Read the model definition and answer for the solid it produces. Units are mm, in the model's axes. Give positions to 0.01 mm unless a question says otherwise; leave off trailing zeros. Order: outer loops, then holes, each group sorted by start corner. A loop starts at its lowest first (then second) coordinate and runs counter-clockwise, first axis right, second up. Notation, with made-up numbers: (78, 32.25) -> (94, 32.25) arc R24 cw to (94, 53.25) -> close; hole circle Ø7 at (-35.75, 72). An arc over 180 degrees is marked (long way). One line per item, written item: value. Start each with the question number.
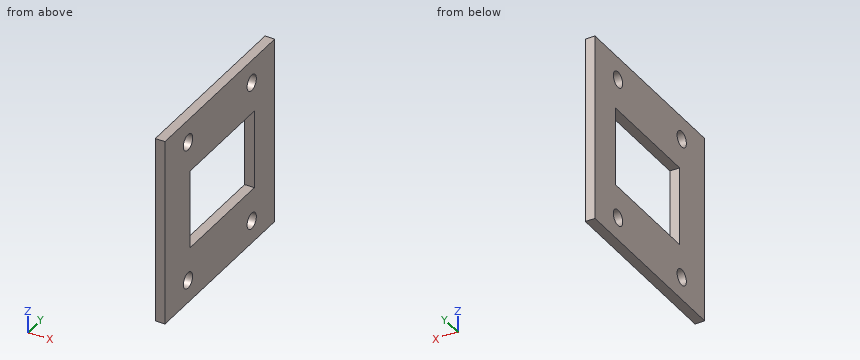
from build123d import *

# Parameters (mm, degrees)
SKETCH1_W           = 61.8
SKETCH1_H           = 62
BOSS_EXTRUDE1_DEPTH = 3.2
CUT_EXTRUDE1_REACH  = 5.2
SKETCH2_W           = 26
SKETCH2_H           = 36.3
CUT_EXTRUDE2_REACH  = 5.2
SKETCH3_R           = 2.625


with BuildPart() as part:
    # Sketch1 → Boss-Extrude1 (new body)
    with BuildSketch(Plane(origin=(0, 0, 0), x_dir=(0, 0, -1), z_dir=(1, 0, 0))):
        with Locations((30.9, 31)):
            Rectangle(SKETCH1_W, SKETCH1_H)
    extrude(amount=BOSS_EXTRUDE1_DEPTH)

    # Sketch2 → Cut-Extrude1 (cut, up to next)
    with BuildSketch(Plane(origin=(3.2, 0, 0), x_dir=(0, 0, -1), z_dir=(1, 0, 0)), mode=Mode.PRIVATE) as cut_extrude1_sk1:
        with Locations((30.9, 32.35)):
            Rectangle(SKETCH2_W, SKETCH2_H)
    cut_extrude1_tool1 = extrude(cut_extrude1_sk1.sketch, amount=-CUT_EXTRUDE1_REACH, mode=Mode.PRIVATE) & part.part
    add(cut_extrude1_tool1.solids().sort_by_distance((3.2, 32.35, -30.9))[0], mode=Mode.SUBTRACT)

    # Sketch3 → Cut-Extrude2 (cut, up to next)
    with BuildSketch(Plane.ZY, mode=Mode.PRIVATE) as cut_extrude2_sk1:
        with Locations((-7.5, 49)):
            Circle(SKETCH3_R)
    cut_extrude2_tool1 = extrude(cut_extrude2_sk1.sketch, amount=-CUT_EXTRUDE2_REACH, mode=Mode.PRIVATE) & part.part
    add(cut_extrude2_tool1.solids().sort_by_distance((0, 49, -7.5))[0], mode=Mode.SUBTRACT)
    # Sketch3 → Cut-Extrude2 (cut, up to next)
    with BuildSketch(Plane.ZY, mode=Mode.PRIVATE) as cut_extrude2_sk2:
        with Locations((-7.5, 13)):
            Circle(SKETCH3_R)
    cut_extrude2_tool2 = extrude(cut_extrude2_sk2.sketch, amount=-CUT_EXTRUDE2_REACH, mode=Mode.PRIVATE) & part.part
    add(cut_extrude2_tool2.solids().sort_by_distance((0, 13, -7.5))[0], mode=Mode.SUBTRACT)
    # Sketch3 → Cut-Extrude2 (cut, up to next)
    with BuildSketch(Plane.ZY, mode=Mode.PRIVATE) as cut_extrude2_sk3:
        with Locations((-54.3, 49)):
            Circle(SKETCH3_R)
    cut_extrude2_tool3 = extrude(cut_extrude2_sk3.sketch, amount=-CUT_EXTRUDE2_REACH, mode=Mode.PRIVATE) & part.part
    add(cut_extrude2_tool3.solids().sort_by_distance((0, 49, -54.3))[0], mode=Mode.SUBTRACT)
    # Sketch3 → Cut-Extrude2 (cut, up to next)
    with BuildSketch(Plane.ZY, mode=Mode.PRIVATE) as cut_extrude2_sk4:
        with Locations((-54.3, 13)):
            Circle(SKETCH3_R)
    cut_extrude2_tool4 = extrude(cut_extrude2_sk4.sketch, amount=-CUT_EXTRUDE2_REACH, mode=Mode.PRIVATE) & part.part
    add(cut_extrude2_tool4.solids().sort_by_distance((0, 13, -54.3))[0], mode=Mode.SUBTRACT)


solid = part.part
Item 1: Find the intervals of material crossed by line 1 (Y direction, x = 1.9, z = -7.5) (3 decimals); line 2 (Y direction, x = 1.15, z = -31); line 3 (Z direction, x = 0.9, y = 36), in increasing order. Write a range as from..to.
Item 2: Find section B-B on y = 13. Write down the section's boundary in (x, z) (3 decimals).
Item 3: Find section C-C on y = 29. Write down the section's boundary in (x, z).
Item 4: Find section D-D on z = -7.5. Write down the section's boundary in (x, y) (3 decimals), then the cut area to 3 significant figures.
Item 5: Find section A-A on z = -34. Write down the section's boundary in (x, y).
Checks:
1. line 1: 0..10.375, 15.625..46.375, 51.625..62
1. line 2: 0..14.2, 50.5..62
1. line 3: -61.8..-43.9, -17.9..0
2. outline: (0, -61.8) -> (3.2, -61.8) -> (3.2, -56.925) -> (0, -56.925) -> close; (0, -51.675) -> (3.2, -51.675) -> (3.2, -10.125) -> (0, -10.125) -> close; (0, -4.875) -> (3.2, -4.875) -> (3.2, 0) -> (0, 0) -> close
3. outline: (0, -61.8) -> (3.2, -61.8) -> (3.2, -43.9) -> (0, -43.9) -> close; (0, -17.9) -> (3.2, -17.9) -> (3.2, 0) -> (0, 0) -> close
4. outline: (0, 0) -> (3.2, 0) -> (3.2, 10.375) -> (0, 10.375) -> close; (0, 15.625) -> (3.2, 15.625) -> (3.2, 46.375) -> (0, 46.375) -> close; (0, 51.625) -> (3.2, 51.625) -> (3.2, 62) -> (0, 62) -> close
4. area: 165 mm2
5. outline: (0, 0) -> (3.2, 0) -> (3.2, 14.2) -> (0, 14.2) -> close; (0, 50.5) -> (3.2, 50.5) -> (3.2, 62) -> (0, 62) -> close
